```python
from build123d import *

# Parameters (mm, degrees)
SKETCH1_W           = 24
SKETCH1_H           = 50
BOSS_EXTRUDE1_DEPTH = 2
SKETCH2_W           = 6
SKETCH2_H           = 40
SKETCH2_W_2         = 9
SKETCH2_H_2         = 10
SKETCH2_W_3         = 5.4
BOSS_EXTRUDE2_DEPTH = 7
FILLET1_R           = 3
SKETCH3_W           = 16.5
SKETCH3_H           = 8
BOSS_EXTRUDE3_DEPTH = 14
SKETCH4_R           = 1.625
CUT_EXTRUDE1_DEPTH  = 45.72135955
CUT_EXTRUDE2_DEPTH  = 2
SKETCH9_W           = 6
SKETCH9_H           = 20
BOSS_EXTRUDE4_DEPTH = 3
SKETCH6_R           = 1.125
CUT_EXTRUDE3_DEPTH  = 39.170669368
SKETCH7_W           = 2
SKETCH7_H           = 40
CUT_EXTRUDE4_DEPTH  = 1
SKETCH8_R           = 1.625
CUT_EXTRUDE5_DEPTH  = 33.015621187
FILLET2_R           = 1
BOSS_EXTRUDE5_DEPTH = 7
LPATTERN1_COUNT     = 5
LPATTERN1_PITCH     = 2


with BuildPart() as part:
    # Sketch1 → Boss-Extrude1 (new body)
    with BuildSketch(Plane(origin=(0, 0, 0), x_dir=(1, 0, 0), z_dir=(0, 1, 0))):
        Rectangle(SKETCH1_W, SKETCH1_H)
    extrude(amount=BOSS_EXTRUDE1_DEPTH)

    # Sketch2 → Boss-Extrude2 (add)
    with BuildSketch(Plane(origin=(0, 2, 0), x_dir=(1, 0, 0), z_dir=(0, 1, 0))):
        with Locations((9, 5)):
            Rectangle(SKETCH2_W, SKETCH2_H)
        with Locations((0, -20)):
            Rectangle(SKETCH2_W_2, SKETCH2_H_2)
        with Locations((-9.3, -20)):
            Rectangle(SKETCH2_W_3, SKETCH2_H_2)
    extrude(amount=BOSS_EXTRUDE2_DEPTH)

    # Fillet1
    fillet1_edges = [part.edges().sort_by_distance(p)[0] for p in [
        (12, 5.5, 15),
        (6, 5.5, 15),
    ]]
    fillet(fillet1_edges, radius=FILLET1_R - 0.0001)  # a hair under: the kernel refuses the full size

    # Sketch3 → Boss-Extrude3 (add)
    with BuildSketch(Plane(origin=(0, 2, 0), x_dir=(1, 0, 0), z_dir=(0, 1, 0))):
        with Locations((3.75, -21)):
            Rectangle(SKETCH3_W, SKETCH3_H)
    extrude(amount=BOSS_EXTRUDE3_DEPTH)

    # Sketch4 → Cut-Extrude1 (cut, through all)
    with BuildSketch(Plane(origin=(0, 0, 15), x_dir=(-1, 0, 0), z_dir=(0, 0, -1))):
        with Locations((0, 5)):
            Circle(SKETCH4_R)
    extrude(amount=-CUT_EXTRUDE1_DEPTH, mode=Mode.SUBTRACT)

    # Sketch5 → Cut-Extrude2 (cut)
    with BuildSketch(Plane(origin=(0, 0, 15), x_dir=(-1, 0, 0), z_dir=(0, 0, -1))):
        Polygon((-2.875, 6.659882024), (-2.875, 9), (2.875, 9), (2.875, 6.659882024), (2.875, 3.340117976), (0, 1.680235952), (-2.875, 3.340117976), align=None)
    extrude(amount=-CUT_EXTRUDE2_DEPTH, mode=Mode.SUBTRACT)

    # Sketch9 → Boss-Extrude4 (add)
    with BuildSketch(Plane(origin=(0, 9, 0), x_dir=(1, 0, 0), z_dir=(0, 1, 0))):
        with Locations((9, -15)):
            Rectangle(SKETCH9_W, SKETCH9_H)
    extrude(amount=BOSS_EXTRUDE4_DEPTH)

    # Sketch6 → Cut-Extrude3 (cut, through all)
    with BuildSketch(Plane(origin=(12, 0, 0), x_dir=(0, 0, -1), z_dir=(1, 0, 0))):
        with Locations((-21, 12.43)):
            Circle(SKETCH6_R)
    extrude(amount=-CUT_EXTRUDE3_DEPTH, mode=Mode.SUBTRACT)

    # Sketch7 → Cut-Extrude4 (cut)
    with BuildSketch(Plane(origin=(0, 2, 0), x_dir=(1, 0, 0), z_dir=(0, 1, 0))):
        with Locations((0, 5)):
            Rectangle(SKETCH7_W, SKETCH7_H)
    extrude(amount=-CUT_EXTRUDE4_DEPTH, mode=Mode.SUBTRACT)

    # Sketch8 → Cut-Extrude5 (cut, through all)
    with BuildSketch(Plane.XZ):
        with Locations(Location((-9, 22, 0), (0, 0, 270))):
            Circle(SKETCH8_R)
        with Locations(Location((9, 10, 0), (0, 0, 270))):
            Circle(SKETCH8_R)
        with Locations(Location((9, -22, 0), (0, 0, 270))):
            Circle(SKETCH8_R)
        with Locations(Location((-9, -22, 0), (0, 0, 270))):
            Circle(SKETCH8_R)
    extrude(amount=-CUT_EXTRUDE5_DEPTH, mode=Mode.SUBTRACT)

    # Fillet2
    fillet2_edges = [part.edges().sort_by_distance(p)[0] for p in [
        (12, 5.5, 17),
        (6, 10.5, 5),
        (12, 10.5, 5),
        (6, 5.5, -25),
        (-4.5, 9, 25),
        (-12, 5.5, 15),
        (-6.6, 5.5, 25),
        (12, 14, 17),
        (-12, 1, -25),
        (12, 4.5, -25),
        (12, 8, 25),
        (-12, 4.5, 25),
    ]]
    fillet(fillet2_edges, radius=FILLET2_R)

    # Sketch10 → Boss-Extrude5 (add)
    with BuildSketch(Plane(origin=(0, 2, 0), x_dir=(1, 0, 0), z_dir=(0, 1, 0))):
        Polygon((-6.6, -24), (-6.6, -23), (-5.85, -23.25), (-5.85, -23.75), align=None)
        Polygon((-5.25, -23.75), (-4.5, -24), (-4.5, -23), (-5.25, -23.25), align=None)
    boss_extrude5 = extrude(amount=BOSS_EXTRUDE5_DEPTH)

    # LPattern1: Boss-Extrude5 ×5
    with Locations(*[(0, 0, -i * LPATTERN1_PITCH) for i in range(1, LPATTERN1_COUNT)]):
        add(boss_extrude5)


solid = part.part
```
For this review, take the finished solid that the model builds, in its own axes (mm). A direction names the side the tool comes from. Round coordinates to 2 decimals unless told otherwise and drop trailing zeros. Loops run counter-clockwise (first coordinate to the right, second up) from the corner with the lowest first, then second, coordinate; pieces in that order, holes last.
(1) Wall thickness on line 1 along X through (y, z) = (0.9, -22) (3 decimals); line 2 along X through (y, z) = (8.75, 10) (3 decimals); line 3 along X through (y, z) = (1.3, -22) (3 decimals): over which ranges is each line inside the solid? List them lowest first.
Returned:
line 1: x = -12 to -10.625, -7.375 to 7.375, 10.625 to 12
line 2: x = 6 to 7.375, 10.625 to 12
line 3: x = -12 to -10.625, -7.375 to -1, 1 to 7.375, 10.625 to 12
(2) We need section B-B (z = 10). Give the boundary of the cut face in (x, y) (3 decimals), plus the area to 3 significant figures.
Returned:
outline: (-12, 0) - (7.375, 0) - (7.375, 12) - (6, 12) - (6, 2) - (1, 2) - (1, 1) - (-1, 1) - (-1, 2) - (-12, 2) - close; (10.625, 0) - (12, 0) - (12, 12) - (10.625, 12) - close
area: 67.0 mm2
(3) We need section D-D (x = -0.5). Give the boundary of the cut face in (y, z) (3 decimals).
Returned:
outline: (0, -25) - (1, -25) - (1, 15) - (1.969, 15) - (1.969, 17) - (3.454, 17) - (3.454, 25) - (0, 25) - close; (6.546, 17) - (16, 17) - (16, 25) - (6.546, 25) - close; hole circle Ø2.25 at (12.43, 21)
(4) We need section C-C (z = -22). Give the boundary of the cut face in (x, y) (3 decimals), plus the area to 4 significant figures.
Returned:
outline: (-12, 0) - (-10.625, 0) - (-10.625, 2) - (-12, 2) - close; (-7.375, 0) - (7.375, 0) - (7.375, 9) - (6, 9) - (6, 2) - (1, 2) - (1, 1) - (-1, 1) - (-1, 2) - (-7.375, 2) - close; (10.625, 0) - (12, 0) - (12, 9) - (10.625, 9) - close
area: 52.25 mm2
(5) Tool access review of faces 1 (the flat face through (-6.6, 5.5, 20.5)), 2 (the flat face through (6, 6, -3)), 3 (the flat face through (9, 10, 5)), 4 (the flat face through (-9, 9, 20)), 5 (the flat face through (9, 9, 16)): name each direction out of +Z, -Z, +X, -X, +Y, -Y from which nothing blocks a thin tool from reaching the whole face with its end or side.
Returned:
face 1: +Y
face 2: -Z, -X, +Y
face 3: -Z, +X, -X, +Y
face 4: +Z, -Z, -X, +Y
face 5: none
(6) Mouldability with a two-part tool opening along Z and no side actions: class faces 6 (the flat face through (-6.6, 5.5, 16.5)), 7 (the cylindrical face through (-11.715, 5.549, 15.301)), 8 (the flat face through (-12, 1, 11)) as released by +Z, released by -Z, zero draft, split by the parting line, or undercut.
Returned:
face 6: undercut
face 7: released by -Z
face 8: zero draft
(7) Clearance check with flat-ended pins moving along their axes: P1, Ø6, axis at y = 3.5, z = 15.5, coming from the +X side; P2, Ø0.5, axis at x = 3.5, z = 16, coming from the +Y side; P3, Ø0.8, axis at y = 4.5, z = 16.5, coming from the +X side; P4, Ø2, axis at x = -4.5, z = 3, coming from the +Y side. State where each tip first meets the part, or that it passes through.
Returned:
P1: stops at x = 12
P2: stops at y = 9
P3: stops at x = 4.5
P4: stops at y = 2
(8) We need section A-A (x = -9). Give the boundary of the cut face in (y, z) (3 decimals), plus the area to 3 significant figures.
Returned:
outline: (0, -25) - (2, -25) - (2, -23.625) - (0, -23.625) - close; (0, -20.375) - (2, -20.375) - (2, 15) - (9, 15) - (9, 20.375) - (0, 20.375) - close; (0, 23.625) - (9, 23.625) - (9, 25) - (0, 25) - close
area: 134 mm2
